Check sheet for the modelled part. Datum: model origin and axes. Units: mm. A direction names the side the tool comes from. Round coordinates to 2 decimals unless told otherwise and drop trailing zeros. Write each loop counter-clockwise with the first axis right and the second up, starting at its lowest first coordinate (ties: lowest second). Pieces come first, ordered by that corner, then holes. Notation, with made-up numbers: M 65,86 L 124,86 A20 cw 124,114 Z; hole C 45.5,26 d11. An arc over 180 degrees is marked long. One line per item, written item: value.
from build123d import *

# Parameters (mm, degrees)
F0_W     = 1065
F0_H     = 1200
F0_W_2   = 1041
F0_H_2   = 1176
F1_DEPTH = 300
F2_W     = 1065
F2_H     = 1200
F3_DEPTH = 12


with BuildPart() as f1:
    # F0 (on Top) → F1 (new body)
    with BuildSketch(Plane.XY):
        Rectangle(F0_W, F0_H)
        Rectangle(F0_W_2, F0_H_2, mode=Mode.SUBTRACT)
    extrude(amount=F1_DEPTH)

    # F2 (on face) → F3 (join)
    with BuildSketch(Plane.XY.offset(300)):
        Rectangle(F2_W, F2_H)
    extrude(amount=-F3_DEPTH)


solid = f1.part
Q1. Sectioned sample at C-C on x = -415.5. Enter the section's corners in (y, z).
Completed:
outline: M -600,0 L -588,0 L -588,288 L 588,288 L 588,0 L 600,0 L 600,300 L -600,300 Z
Q2. Sectioned sample at A-A on z = 205. Enter the section's corners in (x, y).
Completed:
outline: M -532.5,-600 L 532.5,-600 L 532.5,600 L -532.5,600 Z; hole M -520.5,-588 L 520.5,-588 L 520.5,588 L -520.5,588 Z
Q3. Draft check along X on faces 3 (the flat face through (-7, 600, 148)), 4 (the flat face through (532.5, -8, 148)), 5 (the flat face through (520.5, -8, 142)). Enter one of: pulls with the +X half, pulls with the -X half, needs draft (parallel to the pull), parting line crosses it, or undercut.
Completed:
face 3: needs draft
face 4: pulls with the +X half
face 5: undercut
Q4. Scan lines: line 1 (X direction, y = -437.5, z = 78); line 2 (Y direction, x = -252.5, z = 156); line 3 (Z direction, x = -412, y = 48). Record each from-to range of solid material in increasing order. Write a range as [from, to].
Completed:
line 1: [-532.5, -520.5], [520.5, 532.5]
line 2: [-600, -588], [588, 600]
line 3: [288, 300]
Q5. Access from +Z, -Z, +X, -X, +Y, -Y to the whole of each face (thin tool, end or side, straight path). Record for faces 1 (the flat face through (-7, 8, 288)), 2 (the flat face through (-7, -600, 148)).
Completed:
face 1: -Z
face 2: +Z, -Z, +X, -X, -Y
Q6. Sectioned sample at B-B on y = 485.5. Enter the section's corners in (x, z), and give its area (3 significant figures).
Completed:
outline: M -532.5,0 L -520.5,0 L -520.5,288 L 520.5,288 L 520.5,0 L 532.5,0 L 532.5,300 L -532.5,300 Z
area: 19,700 mm^2
